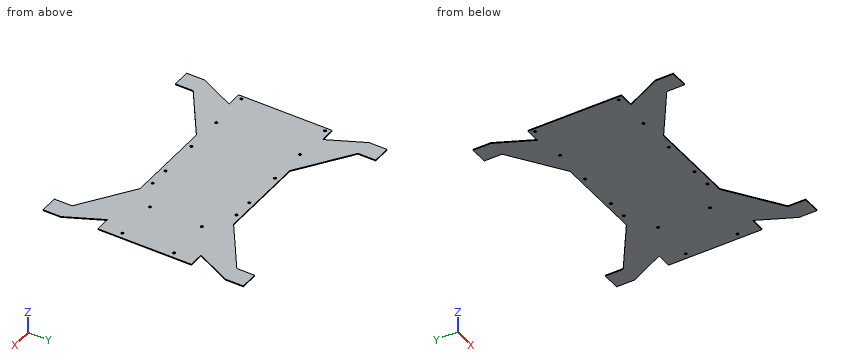
```python
from build123d import *

# Parameters (mm, degrees)
SKETCH_R  = 1.5
PAD_DEPTH = 1


with BuildPart() as part:
    # Sketch → Pad (new body)
    with BuildSketch(Plane.XY):
        Polygon((-125, 52.5), (-108, 52.5), (-127.5, 92.5), (-127.5, 112.5), (-107.5, 112.5), (-107.5, 92.5), (-50, 52.5), (50, 52.5), (107.5, 92.5), (107.5, 112.5), (127.5, 112.5), (127.5, 92.5), (108, 52.5), (125, 52.5), (125, -52.5), (108, -52.5), (127.5, -92.5), (127.5, -112.5), (107.5, -112.5), (107.5, -92.5), (50, -52.5), (-50, -52.5), (-107.5, -92.5), (-107.5, -112.5), (-127.5, -112.5), (-127.5, -92.5), (-108, -52.5), (-125, -52.5), align=None)
        with Locations((-121, -46.965)):
            Circle(SKETCH_R, mode=Mode.SUBTRACT)
        with Locations((-76.58, -46.965)):
            Circle(SKETCH_R, mode=Mode.SUBTRACT)
        with Locations((-32.16, -46.965)):
            Circle(SKETCH_R, mode=Mode.SUBTRACT)
        with Locations((13.54, -46.965)):
            Circle(SKETCH_R, mode=Mode.SUBTRACT)
        with Locations((36.41, -46.965)):
            Circle(SKETCH_R, mode=Mode.SUBTRACT)
        with Locations((36.41, 46.965)):
            Circle(SKETCH_R, mode=Mode.SUBTRACT)
        with Locations((13.54, 46.965)):
            Circle(SKETCH_R, mode=Mode.SUBTRACT)
        with Locations((-32.16, 46.965)):
            Circle(SKETCH_R, mode=Mode.SUBTRACT)
        with Locations((-76.58, 46.965)):
            Circle(SKETCH_R, mode=Mode.SUBTRACT)
        with Locations((-121, 46.965)):
            Circle(SKETCH_R, mode=Mode.SUBTRACT)
        with Locations((69.35627, 29.07)):
            Circle(SKETCH_R, mode=Mode.SUBTRACT)
        with Locations((118.49627, 29.07)):
            Circle(SKETCH_R, mode=Mode.SUBTRACT)
        with Locations((69.35627, -29.07)):
            Circle(SKETCH_R, mode=Mode.SUBTRACT)
        with Locations((118.49627, -29.07)):
            Circle(SKETCH_R, mode=Mode.SUBTRACT)
    extrude(amount=PAD_DEPTH)


solid = part.part
```
Input: part model. Units: mm. Frame: model coordinates. Coordinates: 2 decimals unless noted, no trailing zeros. Order: outer loops, then holes, each group sorted by start corner. A loop starts at its lowest first (then second) coordinate and runs counter-clockwise, first axis right, second up. Notation, with made-up numbers: (47, -9.75) - (54, -9.75) arc R31 ccw to (54, 25.25) - close; hole circle Ø8 at (21, -31). An arc over 180 degrees is marked (long way). Put each result on its own line as item: value.
1. Cut plane B-B on y = 2.5. Return the cut outline in (x, z), then the cut area to 3 significant figures.
Report:
outline: (-125, 0) - (125, 0) - (125, 1) - (-125, 1) - close
area: 250 mm2
2. Cut plane A-A on y = -95.5. Return the cut outline in (x, z).
Report:
outline: (-127.5, 0) - (-107.5, 0) - (-107.5, 1) - (-127.5, 1) - close; (107.5, 0) - (127.5, 0) - (127.5, 1) - (107.5, 1) - close
3. Cut plane C-C on z = 0.85. State how many separate pieces and enclosed holes the cut face has, then the cut area to 3 significant figures.
Report:
separate pieces: 1
enclosed holes: 14
area: 34,000 mm2
4. Contact query for flat-ended pins moving along their axis: pin 1 Ø0.5 at (x, z) = (18, 0.5) entering from +Y; pin 2 Ø0.5 at (y, z) = (8.5, 0.5) entering from +X. Output: stop coordinate, or through.
Report:
pin 1: stops at y = 52.5
pin 2: stops at x = 125
5. Cut plane D-D on x = -55. Return the cut outline in (y, z).
Report:
outline: (-55.98, 0) - (55.98, 0) - (55.98, 1) - (-55.98, 1) - close
6. Line query: line 1 along X through (y, z) = (102, 0.3); line 2 along Y through (x, z) = (13.54, 0.7) (3 decimals); line 3 along Y through (x, z) = (-121, 0.65) (3 decimals). Output: solid intervals per line, ascending.
Report:
line 1: x = -127.5 to -107.5, 107.5 to 127.5
line 2: y = -52.5 to -48.465, -45.465 to 45.465, 48.465 to 52.5
line 3: y = -112.5 to -79.167, -52.5 to -48.465, -45.465 to 45.465, 48.465 to 52.5, 79.167 to 112.5
